Part model, mm, in its own coordinate system. Coordinates: 2 decimals unless noted, no trailing zeros. Loops run counter-clockwise (first coordinate to the right, second up) from the corner with the lowest first, then second, coordinate; pieces in that order, holes last. Notation, with made-up numbers: M 39.5,86 L 82.5,86 A17 ccw 82.5,117 Z; hole C -38,-9 d2. An arc over 180 degrees is marked long. Use a Markdown table: item, result. Add a question column.
1) Band-saw the part on C-C (y = 15). State how many separate pieces and enclosed holes the cut face has, plus the area to 3 significant figures.
2) Pin check, flat tips, straight feed: pin 1 Ø10 at (x, y) = (26.5, 18) entering from +Z; pin 2 Ø1.2 at (x, z) = (58.5, -23) entering from -Y; pin 3 Ø4 at (x, z) = (21.5, -147) entering from -Y. Stop position of each tip, or through.
3) Pull direction Z, two halves, no side cores. Call faces 1 (the flat face through (41, 36, -202)), 2 (the flat face through (0, 36, -102)), 3 (the flat face through (59, 27, -4)): released by +Z, released by -Z, zero draft, split by the parting line, or undercut.
4) Band-saw the part on A-A (z = -179.5). List the corners of the cut face in (x, y).
5) Wall check: probe 1 along Z at (x, y) = (58, 32); probe 2 along X at (y, z) = (27.5, -15); probe 3 along X at (y, z) = (12, -181.5). Give the ranges that are in metal, low to high. Write a range as from..to.
Autodesk Inventor part; units mm, degrees
ref_plane "YZ Plane" through (0, 0, 0) normal (1, 0, 0) x (0, 1, 0)
ref_plane "XZ Plane" through (0, 0, 0) normal (0, 1, 0) x (-1, 0, 0)
ref_plane "XY Plane" through (0, 0, 0) normal (0, 0, 1) x (1, 0, 0)
sketch "Sketch1" plane through (0, 0, 0) normal (0, 1, 0) x (-1, 0, 0)
  line L0 (0, 0) -> (-80, 0)
  line L1 (-80, 0) -> (-80, -202)
  line L2 (-80, -202) -> (0, -202)
  line L3 (0, -202) -> (0, 0)
  line L4 (-4, -4) -> (-38, -4)
  line L5 (-38, -4) -> (-38, -39.6)
  line L6 (-38, -39.6) -> (-4, -39.6)
  line L7 (-4, -39.6) -> (-4, -4)
  line L8 (-4, -43.6) -> (-38, -43.6)
  line L9 (-38, -43.6) -> (-38, -79.2)
  line L10 (-38, -79.2) -> (-4, -79.2)
  line L11 (-4, -79.2) -> (-4, -43.6)
  line L12 (-4, -83.2) -> (-38, -83.2)
  line L13 (-38, -83.2) -> (-38, -118.8)
  line L14 (-38, -118.8) -> (-4, -118.8)
  line L15 (-4, -118.8) -> (-4, -83.2)
  line L16 (-4, -122.8) -> (-38, -122.8)
  line L17 (-38, -122.8) -> (-38, -158.4)
  line L18 (-38, -158.4) -> (-4, -158.4)
  line L19 (-4, -158.4) -> (-4, -122.8)
  line L20 (-42, -158.4) -> (-42, -122.8)
  line L21 (-42, -122.8) -> (-76, -122.8)
  line L22 (-76, -122.8) -> (-76, -158.4)
  line L23 (-76, -158.4) -> (-42, -158.4)
  line L24 (-76, -118.8) -> (-42, -118.8)
  line L25 (-76, -83.2) -> (-76, -118.8)
  line L26 (-42, -118.8) -> (-42, -83.2)
  line L27 (-42, -83.2) -> (-76, -83.2)
  line L28 (-76, -79.2) -> (-42, -79.2)
  line L29 (-76, -43.6) -> (-76, -79.2)
  line L30 (-42, -79.2) -> (-42, -43.6)
  line L31 (-42, -43.6) -> (-76, -43.6)
  line L32 (-76, -39.6) -> (-42, -39.6)
  line L33 (-42, -4) -> (-76, -4)
  line L34 (-42, -39.6) -> (-42, -4)
  line L35 (-76, -4) -> (-76, -39.6)
  line L36 (-4, -162.4) -> (-76, -162.4)
  line L37 (-76, -162.4) -> (-76, -198)
  line L38 (-76, -198) -> (-4, -198)
  line L39 (-4, -198) -> (-4, -162.4)
  point P0 (0, 0)
  dimension "d8" = 34
  dimension "d9" = 35.6
  dimension "d10" = 4
  dimension "d11" = 4
  dimension "d12" = 39.6
  dimension "d20" = 38
  dimension "d25" = 35.6
  dimension "d26" = 4
  dimension "d27" = 4
  dimension "d28" = 4
  dimension "d29" = 4
  dimension "d30" = 4
extrude "Extrusion1" add sketch "Sketch1" along normal blind 70
sketch "Sketch2" plane through (0, 70, 0) normal (0, 1, 0) x (1, 0, 0)
  line L0 (0, 202) -> (0, 0)
  line L1 (0, 0) -> (80, 0)
  line L2 (80, 0) -> (80, 202)
  line L3 (80, 202) -> (0, 202)
extrude "Extrusion2" add sketch "Sketch2" along normal blind 4
fillet "Fillet1" radius 15 36 edges at (76, 70, -180.2) (40, 70, -162.4) (4, 70, -180.2) (40, 70, -198) (76, 70, -21.8) (59, 70, -4) (21, 70, -4) (38, 70, -21.8) (59, 70, -43.6) (76, 70, -61.4) (21, 70, -43.6) (38, 70, -61.4) (21, 70, -83.2) (38, 70, -101) (59, 70, -83.2) (76, 70, -101) (59, 70, -122.8) (76, 70, -140.6) (21, 70, -122.8) (38, 70, -140.6) (4, 70, -21.8) (21, 70, -39.6) (42, 70, -21.8) (59, 70, -39.6) (42, 70, -61.4) (59, 70, -79.2) (4, 70, -61.4) (21, 70, -79.2) (4, 70, -101) (21, 70, -118.8) (42, 70, -101) (59, 70, -118.8) (42, 70, -140.6) (59, 70, -158.4) (4, 70, -140.6) (21, 70, -158.4)
properties part number "Contenedor A" material "ABS Plastic"
Entries:
| question | item | result |
|---|---|---|
| 1 | separate pieces | 1 |
| 1 | enclosed holes | 9 |
| 1 | area | 3,910 mm2 |
| 2 | pin 1 | z = 0 |
| 2 | pin 2 | y = 70 |
| 2 | pin 3 | y = 68.92 |
| 3 | face 1 | released by -Z |
| 3 | face 2 | zero draft |
| 3 | face 3 | undercut |
| 4 | outline | M 0,0 L 4,0 L 4,55 A15 cw 19,70 L 61,70 A15 cw 76,55 L 76,0 L 80,0 L 80,74 L 0,74 Z |
| 5 | probe 1 | -202..-198, -162.4..-158.4, -122.8..-118.8, -83.2..-79.2, -43.6..-39.6, -4..0 |
| 5 | probe 2 | 0..4, 38..42, 76..80 |
| 5 | probe 3 | 0..4, 76..80 |
